```python
from build123d import *

# Parameters (mm, degrees)
SKETCH1_R           = 1.5
SKETCH1_R_2         = 12.5
BOSS_EXTRUDE1_DEPTH = 5
SKETCH2_W           = 20
SKETCH2_H           = 5
BOSS_EXTRUDE2_DEPTH = 25


with BuildPart() as part:
    # Sketch1 → Boss-Extrude1 (new body)
    with BuildSketch(Plane(origin=(0, 0, 0), x_dir=(1, 0, 0), z_dir=(0, 1, 0))):
        with BuildLine():
            Line((-75, -75), (65, -75))
            ThreePointArc((65, -75), (72.071067812, -72.071067812), (75, -65))
            Line((75, -65), (75, 65))
            ThreePointArc((75, 65), (72.071067812, 72.071067812), (65, 75))
            Line((65, 75), (-75, 75))
            Line((-75, 75), (-97.913420794, 18.506857518))
            ThreePointArc((-97.913420794, 18.506857518), (-98.351985938, 17.031769181), (-98.5, 15.5))
            Line((-98.5, 15.5), (-98.5, -15.5))
            ThreePointArc((-98.5, -15.5), (-98.351985938, -17.031769181), (-97.913420794, -18.506857518))
            Line((-97.913420794, -18.506857518), (-75, -75))
        make_face()
        with Locations(Location((-90.5, 15.5, 0), (0, 0, 270))):
            Circle(SKETCH1_R, mode=Mode.SUBTRACT)
        with Locations(Location((-90.5, -15.5, 0), (0, 0, 270))):
            Circle(SKETCH1_R, mode=Mode.SUBTRACT)
        with Locations(Location((-59.5, -15.5, 0), (0, 0, 270))):
            Circle(SKETCH1_R, mode=Mode.SUBTRACT)
        with Locations(Location((-59.5, 15.5, 0), (0, 0, 270))):
            Circle(SKETCH1_R, mode=Mode.SUBTRACT)
        with Locations(Location((-75, 0, 0), (0, 0, 270))):
            Circle(SKETCH1_R_2, mode=Mode.SUBTRACT)
        with Locations(Location((-65, 65, 0), (0, 0, 270))):
            Circle(SKETCH1_R, mode=Mode.SUBTRACT)
        with Locations(Location((65, 65, 0), (0, 0, 270))):
            Circle(SKETCH1_R, mode=Mode.SUBTRACT)
        with Locations(Location((65, -65, 0), (0, 0, 270))):
            Circle(SKETCH1_R, mode=Mode.SUBTRACT)
        with Locations(Location((-65, -65, 0), (0, 0, 270))):
            Circle(SKETCH1_R, mode=Mode.SUBTRACT)
        with Locations(Location((0, 0, 0), (0, 0, 270))):
            Circle(SKETCH1_R, mode=Mode.SUBTRACT)
    extrude(amount=BOSS_EXTRUDE1_DEPTH)

    # Sketch2 → Boss-Extrude2 (add)
    with BuildSketch(Plane(origin=(0, 5, 0), x_dir=(1, 0, 0), z_dir=(0, 1, 0))):
        with Locations((60, 0)):
            Rectangle(SKETCH2_W, SKETCH2_H)
    extrude(amount=-BOSS_EXTRUDE2_DEPTH)


solid = part.part
```
Source: CAD feature listing. Evaluate the final solid. Frame: model axes, mm. A direction names the side the tool comes from. Give positions to 0.01 mm unless a question says otherwise; leave off trailing zeros. Order: outer loops, then holes, each group sorted by start corner. A loop starts at its lowest first (then second) coordinate and runs counter-clockwise, first axis right, second up. Notation, with made-up numbers: (-34, -21) -> (14, -21) arc R31 ccw to (14, 18) -> close; hole circle Ø8 at (-35.75, 17.25). An arc over 180 degrees is marked (long way). Use a Markdown table: item, result.
Q1. First-contact query: P1, Ø4, axis at y = -14, z = 0, coming from the +X side; P2, Ø3.5, axis at x = -90.5, z = -15.5, coming from the -Y side; P3, Ø2.5, axis at x = -65, z = -65, coming from the -Y side; P4, Ø4, axis at x = -59.5, z = -15.5, coming from the +Y side. Flat tips, straight axial feed; report the tip coordinate or a pass-through.
A:
| item | result |
|---|---|
| P1 | x = 70 |
| P2 | y = 0 |
| P3 | through |
| P4 | y = 5 |
Q2. Pull-direction query (Z, two-part tool) for faces 1 (the face through (-62.606, 2.465, -1.627)), 2 (the face through (-86.6, 2.5, 46.4)), 3 (the face through (-13, 0, -1)); classes: +Z half, -Z half, draft (parallel to the pull), parting line (faces both ways), or undercut.
A:
| item | result |
|---|---|
| face 1 | undercut |
| face 2 | +Z half |
| face 3 | draft |
Q3. Section A-A (z = 9.5). Return the cut outline in (x, y).
A:
| item | result |
|---|---|
| outline | (-98.5, 0) -> (-83.12, 0) -> (-83.12, 5) -> (-98.5, 5) -> close; (-66.88, 0) -> (75, 0) -> (75, 5) -> (-66.88, 5) -> close |
Q4. Section B-B (y = -16.5). Return the cut outline in (x, z), and give its area (3 significant figures).
A:
| item | result |
|---|---|
| outline | (50, -2.5) -> (70, -2.5) -> (70, 2.5) -> (50, 2.5) -> close |
| area | 100 mm^2 |
Q5. Access query for faces 4 (the face through (60, -10, 2.5)), 5 (the face through (-86.296, 2.465, -47.149)), 6 (the face through (50, -10, 0)), 7 (the face through (60, -10, -2.5)), 8 (the face through (70, -10, 0)). Directions: +Z, -Z, +X, -X, +Y, -Y. A direction counts if a zero-diameter tool reaches every point of the face in a straight line with its end or side. Return the directions, or none.
A:
| item | result |
|---|---|
| face 4 | +Z, +X, -X, -Y |
| face 5 | -Z, -X, +Y, -Y |
| face 6 | +Z, -Z, -X, -Y |
| face 7 | -Z, +X, -X, -Y |
| face 8 | +Z, -Z, +X, -Y |
Q6. Material intervals for line 1 (X direction, y = 0.25, z = -15.5); line 2 (Z direction, x = 65, y = 2.2); line 3 (X direction, y = 2.7, z = 65), sorted ascending. Write a range as [from, to].
A:
| item | result |
|---|---|
| line 1 | [-98.5, -92], [-89, -61], [-58, 75] |
| line 2 | [-75, -66.5], [-63.5, 63.5], [66.5, 75] |
| line 3 | [-79.06, -66.5], [-63.5, 63.5], [66.5, 75] |
Q7. Section C-C (x = -18.5). Return the cut outline in (y, z).
A:
| item | result |
|---|---|
| outline | (0, -75) -> (5, -75) -> (5, 75) -> (0, 75) -> close |
